Print and shaded views of the part. All mm, measured from the part's lowest x, y and z. Give positions to 0.01 mm unless a question says otherwise; leave off trailing zeros. Loops run counter-clockwise (first coordinate to the right, second up) from the corner with the lowest first, then second, coordinate; pieces in that order, holes last. Notation, with made-up numbers: (-5.75, 67.5) -> (10.25, 67.5) arc R21 cw to (10.25, 102.5) -> close; hole circle Ø6 at (58, -1). An arc over 180 degrees is marked (long way). Answer as a JSON object with one key per item and string values. Group by question number.
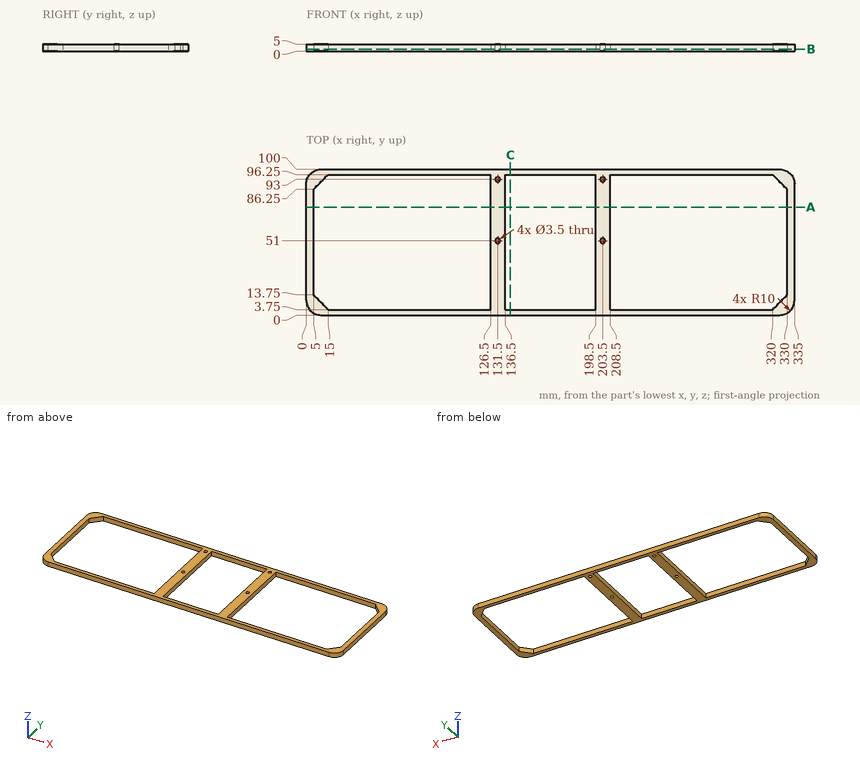
(1) Saw through at A-A on y = 74. List the corners of the cut face in (x, z), plus the area to 3 significant figures.
(2) Saw through at C-C on x = 140. List the corners of the cut face in (y, z).
(3) Saw through at B-B on z = 1.4. List the corners of the cut face in (x, y).
(4) Probe line 1 along X through (y, z) = (24.5, 1.8); line 2 along Y through (x, z) = (131.5, 3.5); line 3 along Y through (x, z) = (195.5, 1.6). List the from-to ranges inside material, lowest first. Write a range as [from, to].
Calculated:
{
 "1": {"outline": "(0, 0) -> (5, 0) -> (5, 5) -> (0, 5) -> close; (126.5, 0) -> (136.5, 0) -> (136.5, 5) -> (126.5, 5) -> close; (198.5, 0) -> (208.5, 0) -> (208.5, 5) -> (198.5, 5) -> close; (330, 0) -> (335, 0) -> (335, 5) -> (330, 5) -> close", "area": "150 mm^2"},
 "2": {"outline": "(0, 0) -> (3.75, 0) -> (3.75, 5) -> (0, 5) -> close; (96.25, 0) -> (100, 0) -> (100, 5) -> (96.25, 5) -> close"},
 "3": {"outline": "(0, 10) arc R10 ccw to (10, 0) -> (325, 0) arc R10 ccw to (335, 10) -> (335, 90) arc R10 ccw to (325, 100) -> (10, 100) arc R10 ccw to (0, 90) -> close; hole (5, 13.75) -> (15, 3.75) -> (126.5, 3.75) -> (126.5, 96.25) -> (15, 96.25) -> (5, 86.25) -> close; hole circle Ø3.5 at (131.5, 51); hole circle Ø3.5 at (131.5, 93); hole (136.5, 3.75) -> (198.5, 3.75) -> (198.5, 96.25) -> (136.5, 96.25) -> close; hole circle Ø3.5 at (203.5, 51); hole circle Ø3.5 at (203.5, 93); hole (208.5, 3.75) -> (320, 3.75) -> (330, 13.75) -> (330, 86.25) -> (320, 96.25) -> (208.5, 96.25) -> close"},
 "4": {"line 1": "x = [0, 5], [126.5, 136.5], [198.5, 208.5], [330, 335]", "line 2": "y = [0, 49.25], [52.75, 91.25], [94.75, 100]", "line 3": "y = [0, 3.75], [96.25, 100]"}
}
